Verification items for the finished model (mm, model axes). Face numbers are marked on the shaded views. A direction names the side the tool comes from. Coordinates: 2 decimals unless noted, no trailing zeros. Order: outer loops, then holes, each group sorted by start corner. A loop starts at its lowest first (then second) coordinate and runs counter-clockwise, first axis right, second up. Notation, with made-up numbers: M -14.75,41.5 L 27.25,41.5 A19 ccw 27.25,73.5 Z; hole C -32.75,16.5 d3. An arc over 180 degrees is marked long. Return JSON: item names as keys, results as strings. Group by question number.
1. Material ranges on line 1 along X through (y, z) = (2.9, -2.5); line 2 along Z through (x, y) = (-10.25, 2.95); line 3 along Z through (x, y) = (-10.5, 1.9), recorded low to high.
2. Section check D-D, the plane y = 3.25. Record the cut outline in (x, z), plus the area to 3 significant figures.
3. Mould release check, pull along Z, two halves, no side actions. Record for the marked faces 1, 2, 3 and 4: +Z half, -Z half, draft (parallel to the pull), parting line (faces both ways), or undercut.
4. Section check B-B, the plane y = 0.5. Record the cut outline in (x, z).
5. Section check C-C, the plane x = -9.5. Record the cut outline in (y, z), plus the area to 3 significant figures.
6. Gauge pin test, flat end, axial feed: pin 1 (3 mm diameter, centred on x = -1, z = 1, fed in from -Y). Record the tip position at first contact, or that the pin passes through.
7. Section check A-A, the plane z = -2.5. Give the number of separate pieces and of enclosed holes in the cut face, plus the area to 3 significant figures.
8. Set-up check for the marked faces 5 and 6: record each of +Z, -Z, +X, -X, +Y, -Y from which the full face is reachable in a straight line by a thin tool's end or side.
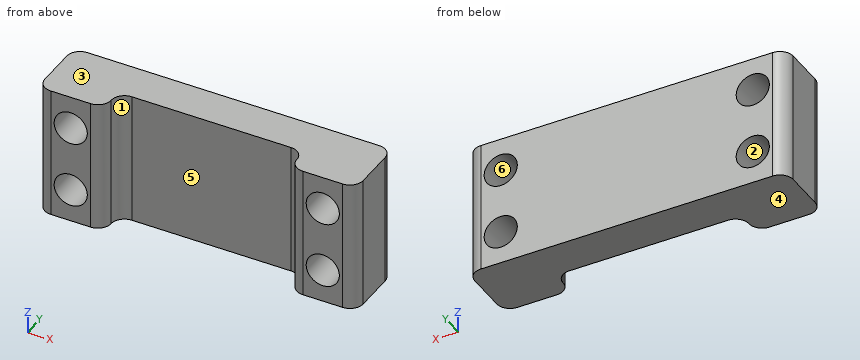
```python
from build123d import *

# Parameters (mm, degrees)
SKETCH1_W           = 24
SKETCH1_H           = 10
BOSS_EXTRUDE1_DEPTH = 5
SKETCH2_W           = 14
SKETCH2_H           = 2
CUT_EXTRUDE1_DEPTH  = 17.401219467
FILLET1_R           = 1
SKETCH3_R           = 1.25
CUT_EXTRUDE2_DEPTH  = 14.928388277


with BuildPart() as part:
    # Sketch1 → Boss-Extrude1 (new body)
    with BuildSketch(Plane(origin=(0, 0, 0), x_dir=(1, 0, 0), z_dir=(0, 1, 0))):
        Rectangle(SKETCH1_W, SKETCH1_H)
    extrude(amount=BOSS_EXTRUDE1_DEPTH)

    # Sketch2 → Cut-Extrude1 (cut, through all)
    with BuildSketch(Plane.XY.offset(5)):
        with Locations((0, 1)):
            Rectangle(SKETCH2_W, SKETCH2_H)
    extrude(amount=-CUT_EXTRUDE1_DEPTH, mode=Mode.SUBTRACT)

    # Fillet1
    fillet1_edges = [part.edges().sort_by_distance(p)[0] for p in [
        (-12, 0, 0),
        (-12, 5, 0),
        (12, 5, 0),
        (12, 0, 0),
        (7, 0, 0),
        (7, 2, 0),
        (-7, 2, 0),
        (-7, 0, 0),
    ]]
    fillet(fillet1_edges, radius=FILLET1_R - 0.0001)  # a hair under: the kernel refuses the full size

    # Sketch3 → Cut-Extrude2 (cut, through all)
    with BuildSketch(Plane(origin=(0, 5, 0), x_dir=(1, 0, 0), z_dir=(0, 1, 0))):
        with Locations(Location((-9.5, 2.5, 0), (0, 0, 270))):
            Circle(SKETCH3_R)
        with Locations(Location((9.5, 2.5, 0), (0, 0, 270))):
            Circle(SKETCH3_R)
        with Locations(Location((-9.5, -2.5, 0), (0, 0, 270))):
            Circle(SKETCH3_R)
        with Locations(Location((9.5, -2.5, 0), (0, 0, 270))):
            Circle(SKETCH3_R)
    extrude(amount=-CUT_EXTRUDE2_DEPTH, mode=Mode.SUBTRACT)


solid = part.part
```
Answers follow:
{
 "1": {"line 1": "-12 to -10.75, -8.25 to 8.25, 10.75 to 12", "line 2": "-5 to -3.5, -1.5 to 1.5, 3.5 to 5", "line 3": "-5 to -3.25, -1.75 to 1.75, 3.25 to 5"},
 "2": {"outline": "M -12,-5 L 12,-5 L 12,5 L -12,5 Z; hole C -9.5,-2.5 d2.5; hole C -9.5,2.5 d2.5; hole C 9.5,-2.5 d2.5; hole C 9.5,2.5 d2.5", "area": "220 mm^2"},
 "3": {"face 1": "draft", "face 2": "undercut", "face 3": "+Z half", "face 4": "-Z half"},
 "4": {"outline": "M -11.87,-5 L -7.13,-5 L -7.13,5 L -11.87,5 Z; M 7.13,-5 L 11.87,-5 L 11.87,5 L 7.13,5 Z; hole C -9.5,-2.5 d2.5; hole C -9.5,2.5 d2.5; hole C 9.5,-2.5 d2.5; hole C 9.5,2.5 d2.5"},
 "5": {"outline": "M 0,-5 L 5,-5 L 5,-3.75 L 0,-3.75 Z; M 0,-1.25 L 5,-1.25 L 5,1.25 L 0,1.25 Z; M 0,3.75 L 5,3.75 L 5,5 L 0,5 Z", "area": "25.0 mm^2"},
 "6": {"pin 1": "y = 2"},
 "7": {"separate pieces": "3", "enclosed holes": "0", "area": "66.1 mm^2"},
 "8": {"face 5": "+Z, -Z, -Y", "face 6": "+Y, -Y"}
}
